Build history of the part. All positions in model axes, mm. Face numbers are marked on the shaded views. A direction names the side the tool comes from. Give positions to 0.01 mm unless a question says otherwise; leave off trailing zeros. Order: outer loops, then holes, each group sorted by start corner. A loop starts at its lowest first (then second) coordinate and runs counter-clockwise, first axis right, second up. Notation, with made-up numbers: (14, 9.25) - (56, 9.25) arc R8 cw to (56, 14.25) - close; hole circle Ø11 at (-22, -15.75). An arc over 180 degrees is marked (long way). One line per item, written item: value.
```python
from build123d import *

# Parameters (mm, degrees)
F0_W        = 1005
F0_H        = 380
F1_DEPTH    = 3.175
F2_W        = 965.2
F2_H        = 330.2
F3_DEPTH    = 76.2
F4_T        = 3.175
F4_T3_DEPTH = 336.55
F4_T5_DEPTH = 971.55
F5_R        = 3.75
F5_R_2      = 12.5
F6_DEPTH    = 3.175
F7_W        = 3.175
F7_H        = 323.85
F8_DEPTH    = 63.5
F10_DEPTH   = 325
F12_DEPTH   = 12.7


# Not quite as in the source:
# - a shell that OpenCascade refuses in one call is made with other operations: the cavity is built on its own and cut out


with BuildPart() as f1:
    # F0 (on Top) → F1 (new body)
    with BuildSketch(Plane.XY):
        Rectangle(F0_W, F0_H)
    extrude(amount=-F1_DEPTH)

    # F2 (on face) → F3 (join)
    with BuildSketch(Plane.XY):
        Rectangle(F2_W, F2_H)
    extrude(amount=F3_DEPTH)

    # F4: shell of thickness 3.175, made by hand


with BuildPart() as f4_core1:
    # F4_t2: copy of F1
    add(f1.part)

    # the walls: a layer under each face that stays
    f4_faces = [f4_core1.faces().sort_by_distance(p)[0] for p in [
        (502.5, 0, -1.5875),
        (0, -190, -1.5875),
        (0, 190, -1.5875),
        (-469, -177.3333333333, 0),
        (0, 0, -3.175),
        (-502.5, 0, -1.5875),
        (482.6, 0, 38.1),
        (0, 165.1, 38.1),
        (-482.6, 0, 38.1),
        (0, -165.1, 38.1),
    ]]
    thicken(f4_faces, amount=-F4_T, mode=Mode.SUBTRACT)

    # F4_s4 → F4_t3 (cut)
    with BuildSketch(Plane.XZ.offset(-168.275)):
        Polygon((482.63175, 0.03175), (482.6, -3.175), (479.425, -3.175), (479.425, 0), align=None)
        Polygon((-482.63175, 0.03175), (-482.6, -3.175), (-479.425, -3.175), (-479.425, 0), align=None)
    extrude(amount=F4_T3_DEPTH, mode=Mode.SUBTRACT)

    # F4_s6 → F4_t5 (cut)
    with BuildSketch(Plane.YZ.offset(-485.775)):
        Polygon((165.13175, 0.03175), (165.1, -3.175), (161.925, -3.175), (161.925, 0), align=None)
        Polygon((-165.13175, 0.03175), (-165.1, -3.175), (-161.925, -3.175), (-161.925, 0), align=None)
    extrude(amount=F4_T5_DEPTH, mode=Mode.SUBTRACT)


with BuildPart() as f1_1:
    add(f1.part)

    # what is left inside the walls is the cavity
    f4_cavity = [f4_core1.part.solids().sort_by_distance(p)[0] for p in [
        (0, -53.975, 0.03175),
    ]]
    add(f4_cavity, mode=Mode.SUBTRACT)

    # F5 (on face) → F6 (cut)
    with BuildSketch(Plane.YZ.offset(482.6)):
        with Locations((-108.1, 38.1)):
            Circle(F5_R)
        with Locations((-38.1, 23.1)):
            Circle(F5_R_2)
        with Locations((31.9, 38.1)):
            Circle(F5_R)
    extrude(amount=-F6_DEPTH, mode=Mode.SUBTRACT)

    # F7 (on face) → F8 (join)
    with BuildSketch(Plane.XY):
        with Locations((122.2375, 0)):
            Rectangle(F7_W, F7_H)
    extrude(amount=F8_DEPTH)

    # F9 (on face) → F10 (join)
    with BuildSketch(Plane(origin=(0, -161.925, 0), x_dir=(-1, 0, 0), z_dir=(0, 1, 0))):
        Polygon((-123.825, 76.2), (-123.825, 63.5), (-120.65, 63.5), (479.425, 63.5), (479.425, 76.2), align=None)
    extrude(amount=F10_DEPTH)

    # F11 (on face) → F12 (cut)
    with BuildSketch(Plane.XY.offset(76.2)):
        with BuildLine():
            ThreePointArc((-457.2, -114.3), (-449.7605122421, -132.2605122421), (-431.8, -139.7))
            Line((-431.8, -139.7), (73.025, -139.7))
            ThreePointArc((73.025, -139.7), (90.9855122421, -132.2605122421), (98.425, -114.3))
            Line((98.425, -114.3), (98.425, 114.3))
            ThreePointArc((98.425, 114.3), (90.9855122421, 132.2605122421), (73.025, 139.7))
            Line((73.025, 139.7), (-431.8, 139.7))
            ThreePointArc((-431.8, 139.7), (-449.7605122421, 132.2605122421), (-457.2, 114.3))
            Line((-457.2, 114.3), (-457.2, -114.3))
        make_face()
    extrude(amount=-F12_DEPTH, mode=Mode.SUBTRACT)


solid = f1_1.part
```
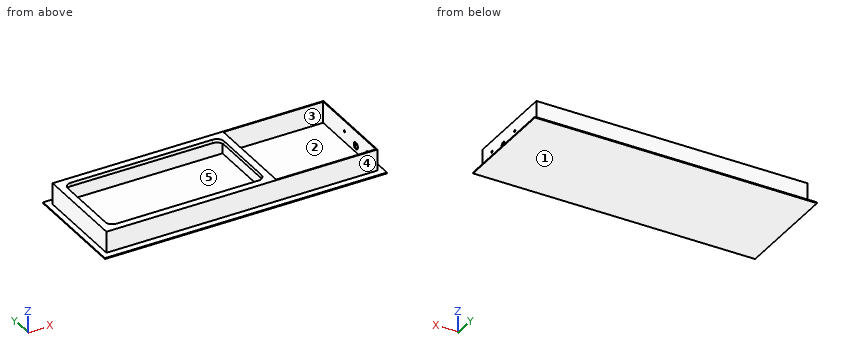
(1) Slice it at A-A, the plane z = 23.1. Give the cut face in (x, y) (3 decimals).
Completed:
outline: (-482.6, -165.1) - (482.6, -165.1) - (482.6, -50.6) - (479.425, -50.6) - (479.425, -161.925) - (123.825, -161.925) - (123.825, 161.925) - (479.425, 161.925) - (479.425, -25.6) - (482.6, -25.6) - (482.6, 165.1) - (-482.6, 165.1) - close; hole (-479.425, -161.925) - (120.65, -161.925) - (120.65, 161.925) - (-479.425, 161.925) - close
(2) Pull direction X, two halves, no side cores. Call the marked faces 1, 2 and 3: +X half, -X half, draft (parallel to the pull), parting line (faces both ways), or undercut.
Completed:
face 1: draft
face 2: undercut
face 3: undercut
(3) Pin check, flat tips, straight feed: P1, Ø10, axis at y = -137.5, z = 21, coming from the -X side; P2, Ø6, axis at x = 322, z = 31, coming from the +Y side; P3, Ø23, axis at y = 1.5, z = 49.5, coming from the +X side. Stop position of each tip, or through.
Completed:
P1: x = -482.6
P2: y = 165.1
P3: x = 482.6
(4) Slice it at C-C, the plane y = 149. Give the cut face in (x, z) (3 decimals), and give its area (3 significant figures).
Completed:
outline: (-502.5, -3.175) - (502.5, -3.175) - (502.5, 0) - (482.6, 0) - (482.6, 76.2) - (479.425, 76.2) - (479.425, 0) - (123.825, 0) - (123.825, 76.2) - (-482.6, 76.2) - (-482.6, 0) - (-502.5, 0) - close; hole (-479.425, 0) - (120.65, 0) - (120.65, 63.5) - (-479.425, 63.5) - close
area: 11,500 mm²
(5) 3-axis set-ups, long thin cutter, end or side, ignore diameter. For the marked faces 4 and 5: which of +Z, -Z, +X, -X, +Y, -Y reach the whole face in a straight line?
Completed:
face 4: +Z, +X, -X, -Y
face 5: none
(6) Slice it at D-D, the plane x = -225.5. Give the cut face in (y, z) (3 decimals).
Completed:
outline: (-190, -3.175) - (190, -3.175) - (190, 0) - (165.1, 0) - (165.1, 76.2) - (139.7, 76.2) - (139.7, 63.5) - (161.925, 63.5) - (161.925, 0) - (-161.925, 0) - (-161.925, 63.5) - (-139.7, 63.5) - (-139.7, 76.2) - (-165.1, 76.2) - (-165.1, 0) - (-190, 0) - close
(7) Slice it at B-B, the plane y = -38.1. Give the cut face in (x, z) (3 decimals), and give its area (3 significant figures).
Completed:
outline: (-502.5, -3.175) - (502.5, -3.175) - (502.5, 0) - (482.6, 0) - (482.6, 10.6) - (479.425, 10.6) - (479.425, 0) - (123.825, 0) - (123.825, 76.2) - (98.425, 76.2) - (98.425, 63.5) - (120.65, 63.5) - (120.65, 0) - (-479.425, 0) - (-479.425, 63.5) - (-457.2, 63.5) - (-457.2, 76.2) - (-482.6, 76.2) - (-482.6, 0) - (-502.5, 0) - close; (479.425, 35.6) - (482.6, 35.6) - (482.6, 76.2) - (479.425, 76.2) - close
area: 4,400 mm²
(8) Drill centre lines: line 1 (X direction, y = 113, z = 45.5) (3 decimals); line 2 (X direction, y = 15, z = 67) (3 decimals); line 3 (Z direction, x = 480, y = 31) (3 decimals). Where is each one in solid material? Low to high.
Completed:
line 1: -482.6 to -479.425, 120.65 to 123.825, 479.425 to 482.6
line 2: -482.6 to -457.2, 98.425 to 123.825, 479.425 to 482.6
line 3: -3.175 to 34.46, 41.74 to 76.2
